Read the model definition and answer for the solid it produces. Units are mm, in the model's axes. A direction names the side the tool comes from. Coordinates: 2 decimals unless noted, no trailing zeros. Write each loop counter-clockwise with the first axis right and the second up, starting at its lowest first coordinate (ties: lowest second). Pieces come first, ordered by that corner, then holes.
(1) Section B-B on y = 9 is taken. State how many separate pieces and enclosed holes the cut face has, then the cut area to 3 significant figures.
(2) Given pin 1 (4 mm diameter, centred on x = -16.25, y = 38.47, fed in from -Z); pin 2 (8 mm diameter, centred on y = 10, z = 28, fed in from +X); pin 3 (13 mm diameter, centred on x = 14.5, z = 42.5, fed in from +Y), each flat-ended and moving along its own axis, determine where each tip first touches the part or whether it passes through.
(3) The mould has two halves that part along X. Classify faces 1 (the flat face through (-22.25, 11, 0)), 2 (the flat face through (-1, 22, 10.5)), 3 (the cylindrical face through (23.65, 21.79, 11.93)), 4 (the flat face through (2, 42, 11)): +X half, -X half, draft (parallel to the pull), parting line (faces both ways), or undercut.
(4) Which of the six approach directions +Z, -Z, +X, -X, +Y, -Y give full straight-line access (tool end or side, diameter ignored) to faces 5 (the conical face through (9.703, 0.285, 49.152)), 6 (the flat face through (-11.15, 9, 0)), 7 (the flat face through (23, 25, 5.5)), 8 (the flat face through (18, 20, 38)), 9 (the conical face through (-23.23, 0.4, -11.5))?
(5) Section D-D on x = 18.5 is taken. Write down the section's boundary in (y, z), then the cut area to 3 significant figures.
(6) Section A-A on x = -16.25 is taken. Write down the section's boundary in (y, z), then the cut area to 3 significant figures.
(7) Section C-C on z = 21 is taken. Write down the section's boundary in (x, y).
(8) Find the intervals of material crossed by probe 1 along X at (y, z) = (2.5, -1); probe 2 along Y at (x, z) = (22.6, 0); probe 3 along Z at (x, y) = (-10, 31), in increasing order.
Autodesk Fusion 360 part; units mm, degrees
sketch "Skizze1" plane through (0, 0, 0) normal (0, 1, 0) x (1, 0, 0)
  line L0 (-24.25, 12.5) -> (24.25, 12.5)
  line L1 (24.25, 12.5) -> (24.25, -12.5)
  line L2 (24.25, -12.5) -> (-24.25, -12.5)
  line L3 (-24.25, -12.5) -> (-24.25, 12.5)
  line L4 (-24.25, 12.5) -> (24.25, -12.5) construction
  line L5 (24.25, 12.5) -> (-24.25, -12.5) construction
  line L6 (22.25, -10.5) -> (-22.25, -10.5)
  line L7 (-22.25, -10.5) -> (-22.25, 10.5)
  line L8 (-22.25, 10.5) -> (22.25, 10.5)
  line L9 (22.25, 10.5) -> (22.25, -10.5)
  line L10 (-22.25, -10.5) -> (-24.25, -10.5)
  line L11 (-22.25, 10.5) -> (-24.25, 10.5)
  dimension "d1" = 48.5
  dimension "d2" = 25
  dimension "d3" = 2
extrude "Extrusion1" add sketch "Skizze1" along normal blind 2 contours L6 L7 L8 L9
extrude "Extrusion3" add sketch "Skizze1" along normal blind 42 contours L0 L1 L2 L3 L6 L8 L9 L10 L11
sketch "Skizze2" plane through (0, 0, 12.5) normal (0, 0, 1) x (1, 0, 0)
  line L0 (-24.25, 0) -> (24.25, 0)
  line L1 (24.25, 0) -> (24.25, 42)
  line L2 (24.25, 42) -> (-24.25, 42)
  line L3 (-24.25, 42) -> (-24.25, 0)
  circle A0 centre (-16.25, 38.4702) radius 1.45
  dimension "d11" = 2.9
sketch "Skizze3" plane through (0, 0, -12.5) normal (0, 0, -1) x (-1, 0, 0)
  line L0 (-24.25, 0) -> (24.25, 0)
  line L1 (24.25, 0) -> (24.25, 42)
  line L2 (24.25, 42) -> (-24.25, 42)
  line L3 (-24.25, 42) -> (-24.25, 0)
  circle A0 centre (16.25, 38.4702) radius 1.45
  dimension "d12" = 2.9
extrude "Extrusion4" cut sketch "Skizze3" against normal blind 2 contours A0
extrude "Extrusion5" cut sketch "Skizze2" against normal blind 2 contours A0
chamfer "Fase1" distance 1.5 angle 45 1 edges at (-17.6019, 38.9946, 12.5)
chamfer "Fase2" distance 1.5 angle 45 1 edges at (-14.8981, 38.9946, -12.5)
sketch "Skizze4" plane through (0, 42, 0) normal (0, 1, 0) x (-1, 0, 0)
  line L0 (-22.25, -10.5) -> (-22.25, 10.5)
  line L1 (-22.25, 10.5) -> (24.25, 10.5)
  line L2 (24.25, 10.5) -> (24.25, 12.5)
  line L3 (24.25, 12.5) -> (-24.25, 12.5)
  line L4 (-24.25, 12.5) -> (-24.25, -12.5)
  line L5 (-24.25, -12.5) -> (24.25, -12.5)
  line L6 (24.25, -12.5) -> (24.25, -10.5)
  line L7 (24.25, -10.5) -> (-22.25, -10.5)
  line L8 (-22.25, -4.75) -> (-24.25, -4.75)
  line L9 (-24.25, -4.75) -> (-24.25, 4.75)
  line L10 (-24.25, 4.75) -> (-22.25, 4.75)
  line L11 (-22.25, 4.75) -> (-22.25, -4.75)
  line L12 (-22.25, -4.75) -> (-24.25, 4.75) construction
  line L13 (-24.25, -4.75) -> (-22.25, 4.75) construction
  point P0 (-23.25, 0)
  dimension "d20" = 2
  dimension "d21" = 9.5
extrude "Extrusion6" add sketch "Skizze4" along normal blind 2.2 contours L0 L4 L8 L9 L10 L11
sketch "Skizze5" plane through (24.25, 0, 0) normal (1, 0, 0) x (0, 0, -1)
  line L0 (-12.5, 0) -> (12.5, 0)
  line L1 (12.5, 0) -> (12.5, 42)
  line L2 (12.5, 42) -> (4.75, 42)
  line L3 (4.75, 42) -> (4.75, 44.2)
  line L4 (4.75, 44.2) -> (-4.75, 44.2)
  line L5 (-4.75, 44.2) -> (-4.75, 42)
  line L6 (-4.75, 42) -> (-12.5, 42)
  line L7 (-12.5, 42) -> (-12.5, 0)
  circle A0 centre (0, 36.7) radius 1.45
  line L8 (5.5, 21.2) -> (-5.5, 21.2)
  line L9 (-5.5, 21.2) -> (-5.5, 28.2)
  line L10 (-5.5, 28.2) -> (5.5, 28.2)
  line L11 (5.5, 28.2) -> (5.5, 21.2)
  line L12 (5.5, 21.2) -> (-5.5, 28.2) construction
  line L13 (-5.5, 21.2) -> (5.5, 28.2) construction
  point P0 (0, 24.7)
  dimension "d25" = 2.9
  dimension "d27" = 11
  dimension "d28" = 7
extrude "Extrusion7" cut sketch "Skizze5" against normal blind 2 contours A0 | L8 L9 L10 L11
chamfer "Fase3" distance 1.5 angle 45 1 edges at (24.25, 37.2243, 1.3519)
extrude "Extrusion8" add sketch "Skizze1" along normal blind 2 contours L3 L7 L10 L11
sketch "Skizze6" plane through (0, 2, 0) normal (0, 1, 0) x (-1, 0, 0)
  line L0 (-22.25, -10.5) -> (24.25, -10.5)
  line L1 (24.25, -10.5) -> (24.25, 10.5)
  line L2 (24.25, 10.5) -> (-22.25, 10.5)
  line L3 (-22.25, 10.5) -> (-22.25, -10.5)
  line L4 (11.15, -10.5) -> (10.35, -10.5)
  line L5 (10.35, -10.5) -> (10.35, 10.5)
  line L6 (10.35, 10.5) -> (11.15, 10.5)
  line L7 (11.15, 10.5) -> (11.15, -10.5)
  line L8 (11.15, -10.5) -> (10.35, 10.5) construction
  line L9 (10.35, -10.5) -> (11.15, 10.5) construction
  line L10 (-6.85, -10.5) -> (-7.65, -10.5)
  line L11 (-7.65, -10.5) -> (-7.65, 10.5)
  line L12 (-7.65, 10.5) -> (-6.85, 10.5)
  line L13 (-6.85, 10.5) -> (-6.85, -10.5)
  line L14 (-6.85, -10.5) -> (-7.65, 10.5) construction
  line L15 (-7.65, -10.5) -> (-6.85, 10.5) construction
  line L16 (-7.65, 10.5) -> (-6.85, 10.5)
  line L17 (-6.85, 10.5) -> (-6.85, 8)
  line L18 (-6.85, 8) -> (-7.65, 8)
  line L19 (-7.65, 8) -> (-7.65, 10.5)
  line L20 (10.35, 10.5) -> (11.15, 10.5)
  line L21 (11.15, 10.5) -> (11.15, 8)
  line L22 (11.15, 8) -> (10.35, 8)
  line L23 (10.35, 8) -> (10.35, 10.5)
  line L24 (-7.65, -10.5) -> (-6.85, -10.5)
  line L25 (-6.85, -10.5) -> (-6.85, -8)
  line L26 (-6.85, -8) -> (-7.65, -8)
  line L27 (-7.65, -8) -> (-7.65, -10.5)
  line L28 (10.35, -10.5) -> (11.15, -10.5)
  line L29 (11.15, -10.5) -> (11.15, -8)
  line L30 (11.15, -8) -> (10.35, -8)
  line L31 (10.35, -8) -> (10.35, -10.5)
  line L32 (-6.85, 0.4172) -> (10.35, 0.4172)
  line L33 (10.35, 0.4172) -> (10.35, -0.3828)
  line L34 (10.35, -0.3828) -> (-6.85, -0.3828)
  line L35 (-6.85, -0.3828) -> (-6.85, 0.4172)
  line L36 (24.25, 10.5) -> (22.25, 10.5)
  line L37 (22.25, 10.5) -> (22.25, -10.5)
  line L38 (22.25, -10.5) -> (24.25, -10.5)
  line L39 (24.25, -10.5) -> (24.25, 10.5)
  point P0 (10.75, 0)
  point P1 (-7.25, 0)
  dimension "d35" = 18
  dimension "d36" = 0.8
  dimension "d37" = 21
  dimension "d38" = 0.8
  dimension "d39" = 21
  dimension "d40" = 0.8
  dimension "d41" = 2.5
  dimension "d42" = 2.5
  dimension "d43" = 2.5
  dimension "d44" = 2.5
  dimension "d49" = 0.8
  dimension "d50" = 2
extrude "Extrusion9" add sketch "Skizze6" along normal blind 10 contours L11 L13 L18 L26 L35 | L5 L7 L22 L30 L33
extrude "Extrusion10" add sketch "Skizze6" along normal blind 19 contours L0 L10 L11 L13 L24 L25 L26 L27 | L2 L11 L12 L13 L16 L17 L18 L19 | L0 L4 L5 L7 L28 L29 L30 L31 | L2 L5 L6 L7 L20 L21 L22 L23
extrude "Extrusion12" add sketch "Skizze6" along normal blind 19 contours L0 L1 L2 L36 L37 L38 L39
extrude "Extrusion13" add sketch "Skizze6" along normal blind 8 contours L5 L13 L32 L33 L34 L35
chamfer "Fase4" distance 1 angle 45 4 edges at (-10.75, 21, 8) (7.25, 21, 8) (-10.75, 21, -8) (7.25, 21, -8)
fillet "Abrundung1" radius 2 2 edges at (24.25, 21, -12.5) (24.25, 21, 12.5)
fillet "Abrundung2" radius 0.5 2 edges at (22.25, 22, 10.5) (22.25, 22, -10.5)
fillet "Abrundung3" radius 2 2 edges at (-24.25, 21, 12.5) (-24.25, 21, -12.5)
sketch "Skizze8" plane through (0, 0, 12.5) normal (0, 0, 1) x (1, 0, 0)
  line L0 (-22.25, 42) -> (-22.25, 0)
  line L1 (-22.25, 0) -> (22.25, 0)
  line L2 (22.25, 0) -> (22.25, 42)
  line L3 (22.25, 42) -> (-22.25, 42)
  circle A0 centre (-16.25, 38.4702) radius 2.95
  line L4 (22, 0) -> (16, 0)
  line L5 (16, 0) -> (16, 20)
  line L6 (16, 20) -> (22, 20)
  line L7 (22, 20) -> (22, 0)
  line L8 (22, 0) -> (16, 20) construction
  line L9 (16, 0) -> (22, 20) construction
  point P0 (19, 10)
  dimension "d68" = 6
  dimension "d69" = 20
extrude "Extrusion15" add sketch "Skizze8" along normal blind 43 contours L1 L4 L5 L6 L7
sketch "Skizze9" plane through (16, 0, 0) normal (-1, 0, 0) x (0, 0, 1)
  line L0 (12.5, 20) -> (12.5, 0)
  line L1 (12.5, 0) -> (55.5, 0)
  line L2 (55.5, 0) -> (55.5, 20)
  line L3 (55.5, 20) -> (12.5, 20)
  line L4 (55.5, 20) -> (47.5, 20)
  line L5 (47.5, 20) -> (47.5, 0)
  line L6 (47.5, 0) -> (55.5, 0)
  line L7 (55.5, 0) -> (55.5, 20)
  dimension "d72" = 8
extrude "Extrusion16" add sketch "Skizze9" along normal blind 8 contours L1 L2 L3 L4 L5 L6 L7
sketch "Skizze10" plane through (0, 0, 0) normal (0, -1, 0) x (1, 0, 0)
  line L0 (8, 47.5) -> (16, 47.5)
  line L1 (16, 47.5) -> (16, 12.5)
  line L2 (22.25, 12.5) -> (22, 12.5)
  arc A0 (-22.25, 12.5) -> (-24.25, 10.5) centre (-22.25, 10.5) ccw
  line L3 (-24.25, 10.5) -> (-24.25, -10.5)
  arc A1 (-24.25, -10.5) -> (-22.25, -12.5) centre (-22.25, -10.5) ccw
  line L4 (-22.25, -12.5) -> (22.25, -12.5)
  arc A2 (22.25, -12.5) -> (24.25, -10.5) centre (22.25, -10.5) ccw
  line L5 (24.25, -10.5) -> (24.25, 10.5)
  arc A3 (24.25, 10.5) -> (22.25, 12.5) centre (22.25, 10.5) ccw
  line L6 (22, 12.5) -> (22, 55.5)
  line L7 (22, 55.5) -> (8, 55.5)
  circle A4 centre (11.5, 51.5) radius 1.75
  line L8 (8, 55.5) -> (8, 47.5)
  line L9 (16, 12.5) -> (-22.25, 12.5)
  dimension "d77" = 3.5
extrude "Extrusion17" cut sketch "Skizze10" against normal blind 20 contours A4
sketch "Skizze11" plane through (8, 0, 0) normal (-1, 0, 0) x (0, 0, 1)
  line L0 (55.5, 0) -> (55.5, 20)
  line L1 (55.5, 20) -> (47.5, 20)
  line L2 (47.5, 20) -> (47.5, 0)
  line L3 (47.5, 0) -> (55.5, 0)
  line L4 (55.5, 6.25) -> (47.5, 6.25)
  line L5 (47.5, 6.25) -> (47.5, 13.75)
  line L6 (47.5, 13.75) -> (55.5, 13.75)
  line L7 (55.5, 13.75) -> (55.5, 6.25)
  line L8 (55.5, 6.25) -> (47.5, 13.75) construction
  line L9 (47.5, 6.25) -> (55.5, 13.75) construction
  point P0 (51.5, 10)
  dimension "d80" = 7.5
extrude "Extrusion18" cut sketch "Skizze11" against normal blind 8 contours L0 L2 L4 L5 L6 L7
fillet "Abrundung5" radius 4 4 edges at (8, 16.875, 47.5) (8, 16.875, 55.5) (8, 3.125, 47.5) (8, 3.125, 55.5)
chamfer "Fase10" distance 1 angle 45 19 edges at (14, 0, 47.5) (8, 0, 51.5) (17, 0, 55.5) (22, 0, 34) (23.6642, 0, 11.9142) (24.25, 0, 0) (23.6642, 0, -11.9142) (0, 0, -12.5) (-23.6642, 0, -11.9142) (-24.25, 0, 0) (-23.6642, 0, 11.9142) (-3.125, 0, 12.5) (22.125, 0, 12.5) (16, 0, 30) (22, 20, 34) (17, 20, 55.5) (8, 20, 51.5) (14, 20, 47.5) (16, 20, 30)
chamfer "Fase11" distance 1 angle 45 1 edges at (22, 10, 55.5)
Response:
1. separate pieces: 1
1. enclosed holes: 4
1. area: 580 mm2
2. pin 1: stops at z = -11.55
2. pin 2: stops at x = 22
2. pin 3: stops at y = 20
3. face 1: undercut
3. face 2: undercut
3. face 3: +X half
3. face 4: draft
4. face 5: -X, -Y
4. face 6: +Y
4. face 7: +X, -X
4. face 8: +Z, +X, -X, +Y
4. face 9: -Z, -X, -Y
5. outline: (0, -11.5) - (1, -12.5) - (42, -12.5) - (42, -10.5) - (2, -10.5) - (2, 10.5) - (42, 10.5) - (42, 12.5) - (20, 12.5) - (20, 54.5) - (19, 55.5) - (1, 55.5) - (0, 54.5) - close
5. area: 1,070 mm2
6. outline: (0, -11.5) - (1, -12.5) - (35.52, -12.5) - (37.02, -11) - (37.02, -10.5) - (2, -10.5) - (2, 10.5) - (37.02, 10.5) - (37.02, 11) - (35.52, 12.5) - (1, 12.5) - (0, 11.5) - close; (39.92, -11) - (41.42, -12.5) - (42, -12.5) - (42, -10.5) - (39.92, -10.5) - close; (39.92, 10.5) - (42, 10.5) - (42, 12.5) - (41.42, 12.5) - (39.92, 11) - close
6. area: 193 mm2
7. outline: (16, 1) - (17, 0) - (21, 0) - (22, 1) - (22, 19) - (21, 20) - (17, 20) - (16, 19) - close
8. probe 1: x = -24.25 to -22.25, -11.15 to -10.35, 6.85 to 7.65, 22.25 to 24.25
8. probe 2: y = 0 to 21.2, 28.2 to 35.25, 38.15 to 44.2
8. probe 3: z = -12.5 to -10.5, 10.5 to 12.5
